Verification items for the finished model (mm, model axes). A direction names the side the tool comes from. Coordinates: 2 decimals unless noted, no trailing zeros. Order: outer loops, then holes, each group sorted by start corner. A loop starts at its lowest first (then second) coordinate and runs counter-clockwise, first axis right, second up. Notation, with made-up numbers: (17, -12.5) -> (59, -12.5) arc R20 cw to (59, -4.5) -> close; hole circle Ø8 at (50, -8.5). An arc over 180 degrees is marked (long way). Use CSV: the item, a comma, the result in double quotes. Start each with the question number.
1) Sectioned sample at B-B on y = 3.5. Give the number of separate pieces and of enclosed holes in the cut face, then the cut area to 3 significant figures.
2) Go/stop test with flat-tipped pins: pin 1 (1.5 mm diameter, centred on x = 748.5, y = 5, fed in from -Z); pin 2 (0.5 mm diameter, centred on x = 691.5, y = 6.5, fed in from -Z). Record where each tip stops, or that it passes through.
3) Sectioned sample at A-A on z = -168.5. Record the boundary of the cut face in (x, y) (3 decimals), then the cut area to 3 significant figures.
4) Scan lines: line 1 along X through (y, z) = (3.5, -361.95); line 2 along X through (y, z) = (4.5, -361); line 3 along X through (y, z) = (2.5, -298). Record each from-to range of solid material in increasing order.
5) Sectioned sample at C-C on x = 102.5. Record the boundary of the cut face in (y, z) (3 decimals), then the cut area to 3 significant figures.
6) Release check for a two-part mould opening along X. For faces 3 (the cylindrical face through (995.66, 4.7, -38.99)), 4 (the flat face through (536, 0, -22)) record: released by +X, released by -X, zero draft, split by the parting line, or undercut.
7) Tool access check on faces 1 (the flat face through (536, 9.525, -22)), 2 (the cylindrical face through (70.74, 4.7, -39.39)). Record the directions out of +Z, -Z, +X, -X, +Y, -Y that give a thin tool (end or side, any length) a straight path to the whole face; none if there is none.
8) Sectioned sample at D-D on x = 673.5. Record the boundary of the cut face in (y, z) (3 decimals).
from build123d import *

# Parameters (mm, degrees)
SKETCH1_R           = 3.3734375
BOSS_EXTRUDE1_DEPTH = 9.525


with BuildPart() as part:
    # Sketch1 → Boss-Extrude1 (new body)
    with BuildSketch(Plane(origin=(0, 0, 0), x_dir=(1, 0, 0), z_dir=(0, 1, 0))):
        with BuildLine():
            Line((1006.475, 384.175), (1063.625, 384.175))
            ThreePointArc((1063.625, 384.175), (1065.87006403, 383.24506403), (1066.8, 381))
            Line((1066.8, 381), (1066.8, 3.175))
            ThreePointArc((1066.8, 3.175), (1065.87006403, 0.92993597), (1063.625, 0))
            Line((1063.625, 0), (3.175, 0))
            ThreePointArc((3.175, 0), (0.92993597, 0.92993597), (0, 3.175))
            Line((0, 3.175), (0, 381))
            ThreePointArc((0, 381), (0.92993597, 383.24506403), (3.175, 384.175))
            Line((3.175, 384.175), (60.325, 384.175))
            ThreePointArc((60.325, 384.175), (62.57006403, 383.24506403), (63.5, 381))
            Line((63.5, 381), (63.5, 342.9))
            ThreePointArc((63.5, 342.9), (62.57006403, 340.65493597), (60.325, 339.725))
            Line((60.325, 339.725), (34.925, 339.725))
            ThreePointArc((34.925, 339.725), (32.67993597, 338.79506403), (31.75, 336.55))
            Line((31.75, 336.55), (31.75, 73.025))
            ThreePointArc((31.75, 73.025), (32.67993597, 70.77993597), (34.925, 69.85))
            Line((34.925, 69.85), (60.325, 69.85))
            ThreePointArc((60.325, 69.85), (62.57006403, 68.92006403), (63.5, 66.675))
            Line((63.5, 66.675), (63.5, 57.15))
            ThreePointArc((63.5, 57.15), (70.939487758, 39.189487758), (88.9, 31.75))
            Line((88.9, 31.75), (346.075, 31.75))
            ThreePointArc((346.075, 31.75), (364.035512242, 39.189487758), (371.475, 57.15))
            Line((371.475, 57.15), (371.475, 60.325))
            ThreePointArc((371.475, 60.325), (372.40493597, 62.57006403), (374.65, 63.5))
            Line((374.65, 63.5), (376.2375, 63.5))
            ThreePointArc((376.2375, 63.5), (378.48256403, 62.57006403), (379.4125, 60.325))
            Line((379.4125, 60.325), (379.4125, 57.15))
            ThreePointArc((379.4125, 57.15), (386.851987758, 39.189487758), (404.8125, 31.75))
            Line((404.8125, 31.75), (661.9875, 31.75))
            ThreePointArc((661.9875, 31.75), (679.948012242, 39.189487758), (687.3875, 57.15))
            Line((687.3875, 57.15), (687.3875, 60.325))
            ThreePointArc((687.3875, 60.325), (688.31743597, 62.57006403), (690.5625, 63.5))
            Line((690.5625, 63.5), (692.15, 63.5))
            ThreePointArc((692.15, 63.5), (694.39506403, 62.57006403), (695.325, 60.325))
            Line((695.325, 60.325), (695.325, 57.15))
            ThreePointArc((695.325, 57.15), (702.764487758, 39.189487758), (720.725, 31.75))
            Line((720.725, 31.75), (977.9, 31.75))
            ThreePointArc((977.9, 31.75), (995.860512242, 39.189487758), (1003.3, 57.15))
            Line((1003.3, 57.15), (1003.3, 66.675))
            ThreePointArc((1003.3, 66.675), (1004.22993597, 68.92006403), (1006.475, 69.85))
            Line((1006.475, 69.85), (1031.875, 69.85))
            ThreePointArc((1031.875, 69.85), (1034.12006403, 70.77993597), (1035.05, 73.025))
            Line((1035.05, 73.025), (1035.05, 336.55))
            ThreePointArc((1035.05, 336.55), (1034.12006403, 338.79506403), (1031.875, 339.725))
            Line((1031.875, 339.725), (1006.475, 339.725))
            ThreePointArc((1006.475, 339.725), (1004.22993597, 340.65493597), (1003.3, 342.9))
            Line((1003.3, 342.9), (1003.3, 381))
            ThreePointArc((1003.3, 381), (1004.22993597, 383.24506403), (1006.475, 384.175))
        make_face()
        with Locations(Location((22.225, 361.95, 0), (0, 0, 90))):
            Circle(SKETCH1_R, mode=Mode.SUBTRACT)
        with Locations(Location((1044.575, 361.95, 0), (0, 0, 90))):
            Circle(SKETCH1_R, mode=Mode.SUBTRACT)
    extrude(amount=BOSS_EXTRUDE1_DEPTH)


solid = part.part
Answers follow:
1,separate pieces,"1"
1,enclosed holes,"2"
1,area,"62,700 mm²"
2,pin 1,"stops at z = -31.75"
2,pin 2,"stops at z = -63.5"
3,outline,"(0, 0) -> (31.75, 0) -> (31.75, 9.525) -> (0, 9.525) -> close; (1035.05, 0) -> (1066.8, 0) -> (1066.8, 9.525) -> (1035.05, 9.525) -> close"
3,area,"605 mm²"
4,line 1,"x = 0 to 18.85, 25.6 to 63.5, 1003.3 to 1041.2, 1047.95 to 1066.8"
4,line 2,"x = 0 to 18.99, 25.46 to 63.5, 1003.3 to 1041.34, 1047.81 to 1066.8"
4,line 3,"x = 0 to 31.75, 1035.05 to 1066.8"
5,outline,"(0, -31.75) -> (9.525, -31.75) -> (9.525, 0) -> (0, 0) -> close"
5,area,"302 mm²"
6,face 3,"undercut"
6,face 4,"zero draft"
7,face 1,"+Z, -Z, +X, -X, +Y"
7,face 2,"-Z, +Y, -Y"
8,outline,"(0, -34.509) -> (9.525, -34.509) -> (9.525, 0) -> (0, 0) -> close"
